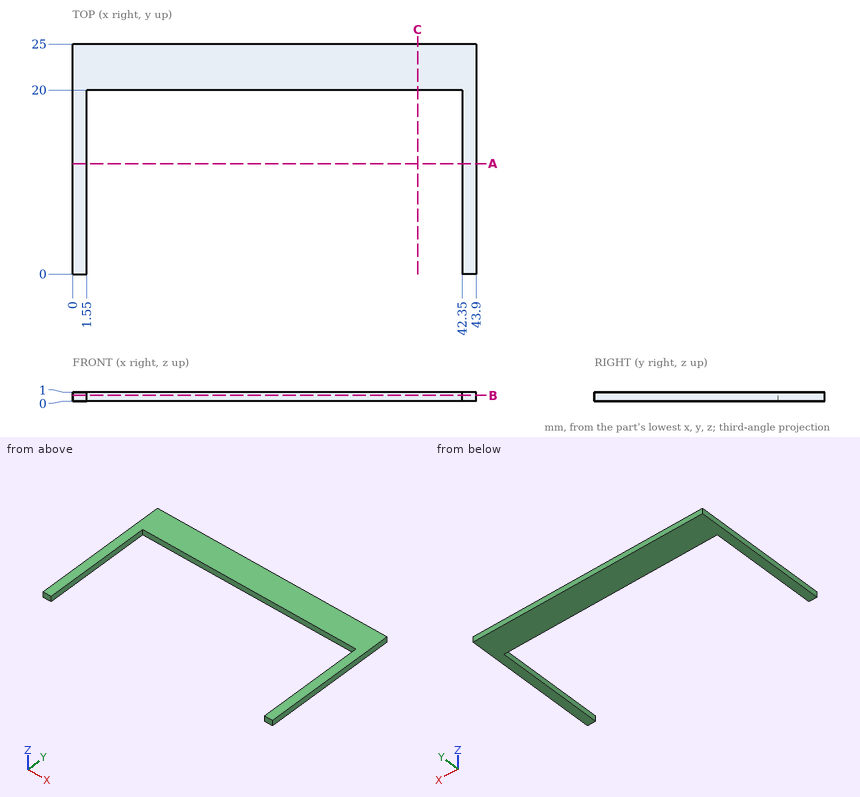
Check sheet for the drawn part. Datum: minimum x, y, z corner. Units: mm. Give positions to 0.01 mm unless a question says otherwise; leave off trailing zeros. Order: outer loops, then holes, each group sorted by start corner. A loop starts at its lowest first (then second) coordinate and runs counter-clockwise, first axis right, second up. Notation, with made-up numbers: (-19, 50.5) - (36, 50.5) arc R21 ccw to (36, 58.5) - close; hole circle Ø6 at (23, 9.25). An arc over 180 degrees is marked (long way). Write item = value, one per line. Start each with the question number.
1) Gauge pin test, flat ends, axial feed: pin 1 Ø6 at (x, y) = (32.5, 15.5) entering from +Z (1 decimal); pin 2 Ø0.5 at (x, z) = (25, 0.5) entering from -Y. Record the tip position at first contact, or that the pin passes through.
2) Scan lines: L1, parallel to X at y = 11, z = 0.6; L2, parallel to Y at x = 37, z = 0.4. Record each from-to range of solid material in increasing order.
3) Section check A-A (y = 12). Enter the section's corners in (x, z).
4) Section check B-B (z = 0.65). Enter the section's corners in (x, y).
5) Section check C-C (x = 37.5). Enter the section's corners in (y, z), then the cut area to 3 significant figures.
Geometry check:
q1.pin_1 = through
q1.pin_2 = 20
q2.L1 = 0 to 1.55, 42.35 to 43.9
q2.L2 = 20 to 25
q3.outline = (0, 0) - (1.55, 0) - (1.55, 1) - (0, 1) - close; (42.35, 0) - (43.9, 0) - (43.9, 1) - (42.35, 1) - close
q4.outline = (0, 0) - (1.55, 0) - (1.55, 20) - (42.35, 20) - (42.35, 0) - (43.9, 0) - (43.9, 25) - (0, 25) - close
q5.outline = (20, 0) - (25, 0) - (25, 1) - (20, 1) - close
q5.area = 5.00 mm2
